Read the model definition and answer for the solid it produces. Units are mm, in the model's axes. A direction names the side the tool comes from. Round coordinates to 2 decimals unless told otherwise and drop trailing zeros. Loops run counter-clockwise (first coordinate to the right, second up) from the corner with the lowest first, then second, coordinate; pieces in that order, holes last. Notation, with made-up numbers: (-13.5, 25.5) - (-7.5, 25.5) arc R9 ccw to (-7.5, 40.5) - close; hole circle Ø8 at (73.25, 39.5). An arc over 180 degrees is marked (long way). Use one line per item in the form item = value. Start each with the question number.
```python
from build123d import *

# Parameters (mm, degrees)
SKETCH1_R           = 3.175
SKETCH1_R_2         = 2.54
BOSS_EXTRUDE1_DEPTH = 3.175
SKETCH2_R           = 11.049
SKETCH2_R_2         = 15.875
SKETCH2_R_3         = 1.27
CUT_EXTRUDE1_DEPTH  = 205.928972451


with BuildPart() as part:
    # Sketch1 → Boss-Extrude1 (new, symmetric)
    with BuildSketch(Plane.XY):
        with BuildLine():
            Line((-83.815331135, 50.8), (83.815331135, 50.8))
            ThreePointArc((83.815331135, 50.8), (193.675, 0), (83.815331135, -50.8))
            Line((83.815331135, -50.8), (-83.815331135, -50.8))
            ThreePointArc((-83.815331135, -50.8), (-193.675, 0), (-83.815331135, 50.8))
        make_face()
        with Locations((-127, 0)):
            Circle(SKETCH1_R, mode=Mode.SUBTRACT)
        with Locations((127, 0)):
            Circle(SKETCH1_R, mode=Mode.SUBTRACT)
        with Locations((-127, 57.15)):
            Circle(SKETCH1_R_2, mode=Mode.SUBTRACT)
        with Locations((-86.588847455, 40.411152545)):
            Circle(SKETCH1_R_2, mode=Mode.SUBTRACT)
        with Locations((-69.85, 0)):
            Circle(SKETCH1_R_2, mode=Mode.SUBTRACT)
        with Locations((-86.588847455, -40.411152545)):
            Circle(SKETCH1_R_2, mode=Mode.SUBTRACT)
        with Locations((-127, -57.15)):
            Circle(SKETCH1_R_2, mode=Mode.SUBTRACT)
        with Locations((-167.411152545, -40.411152545)):
            Circle(SKETCH1_R_2, mode=Mode.SUBTRACT)
        with Locations((-167.411152545, 40.411152545)):
            Circle(SKETCH1_R_2, mode=Mode.SUBTRACT)
        with Locations(Location((127, 57.15, 0), (0, 0, 180))):
            Circle(SKETCH1_R_2, mode=Mode.SUBTRACT)
        with Locations(Location((167.411152545, 40.411152545, 0), (0, 0, 180))):
            Circle(SKETCH1_R_2, mode=Mode.SUBTRACT)
        with Locations(Location((167.411152545, -40.411152545, 0), (0, 0, 180))):
            Circle(SKETCH1_R_2, mode=Mode.SUBTRACT)
        with Locations(Location((127, -57.15, 0), (0, 0, 180))):
            Circle(SKETCH1_R_2, mode=Mode.SUBTRACT)
        with Locations(Location((86.588847455, -40.411152545, 0), (0, 0, 180))):
            Circle(SKETCH1_R_2, mode=Mode.SUBTRACT)
        with Locations(Location((69.85, 0, 0), (0, 0, 180))):
            Circle(SKETCH1_R_2, mode=Mode.SUBTRACT)
        with Locations(Location((86.588847455, 40.411152545, 0), (0, 0, 180))):
            Circle(SKETCH1_R_2, mode=Mode.SUBTRACT)
    extrude(amount=BOSS_EXTRUDE1_DEPTH, both=True)

    # Sketch2 → Cut-Extrude1 (cut, through all)
    with BuildSketch(Plane.XY.offset(3.175)):
        with Locations((-127, 0)):
            Circle(SKETCH2_R)
        with Locations((-155.575, 0)):
            Circle(SKETCH2_R_2)
        with Locations((-155.575, 23.8125)):
            Circle(SKETCH2_R_3)
        with Locations((-138.737019773, 16.837980227)):
            Circle(SKETCH2_R_3)
        with Locations((-138.737019773, -16.837980227)):
            Circle(SKETCH2_R_3)
        with Locations((-155.575, -23.8125)):
            Circle(SKETCH2_R_3)
        with Locations((-172.412980227, -16.837980227)):
            Circle(SKETCH2_R_3)
        with Locations((-179.3875, 0)):
            Circle(SKETCH2_R_3)
        with Locations((-172.412980227, 16.837980227)):
            Circle(SKETCH2_R_3)
        with Locations((-127, 15.875)):
            Circle(SKETCH2_R_3)
        with Locations((-115.774679849, 11.225320151)):
            Circle(SKETCH2_R_3)
        with Locations((-111.125, 0)):
            Circle(SKETCH2_R_3)
        with Locations((-115.774679849, -11.225320151)):
            Circle(SKETCH2_R_3)
        with Locations((-127, -15.875)):
            Circle(SKETCH2_R_3)
        with Locations((-138.225320151, -11.225320151)):
            Circle(SKETCH2_R_3)
        with Locations(Location((138.225320151, 11.225320151, 0), (0, 0, 180))):
            Circle(SKETCH2_R_3)
        with Locations((-138.225320151, 11.225320151)):
            Circle(SKETCH2_R_3)
        with Locations(Location((138.225320151, -11.225320151, 0), (0, 0, 180))):
            Circle(SKETCH2_R_3)
        with Locations(Location((127, -15.875, 0), (0, 0, 180))):
            Circle(SKETCH2_R_3)
        with Locations(Location((115.774679849, -11.225320151, 0), (0, 0, 180))):
            Circle(SKETCH2_R_3)
        with Locations(Location((111.125, 0, 0), (0, 0, 180))):
            Circle(SKETCH2_R_3)
        with Locations(Location((115.774679849, 11.225320151, 0), (0, 0, 180))):
            Circle(SKETCH2_R_3)
        with Locations(Location((127, 15.875, 0), (0, 0, 180))):
            Circle(SKETCH2_R_3)
        with Locations(Location((172.412980227, 16.837980227, 0), (0, 0, 180))):
            Circle(SKETCH2_R_3)
        with Locations(Location((179.3875, 0, 0), (0, 0, 180))):
            Circle(SKETCH2_R_3)
        with Locations(Location((172.412980227, -16.837980227, 0), (0, 0, 180))):
            Circle(SKETCH2_R_3)
        with Locations(Location((155.575, -23.8125, 0), (0, 0, 180))):
            Circle(SKETCH2_R_3)
        with Locations(Location((138.737019773, -16.837980227, 0), (0, 0, 180))):
            Circle(SKETCH2_R_3)
        with Locations(Location((138.737019773, 16.837980227, 0), (0, 0, 180))):
            Circle(SKETCH2_R_3)
        with Locations(Location((155.575, 23.8125, 0), (0, 0, 180))):
            Circle(SKETCH2_R_3)
        with Locations(Location((155.575, 0, 0), (0, 0, 180))):
            Circle(SKETCH2_R_2)
        with Locations(Location((127, 0, 0), (0, 0, 180))):
            Circle(SKETCH2_R)
    extrude(amount=-CUT_EXTRUDE1_DEPTH, mode=Mode.SUBTRACT)


solid = part.part
```
1) A cutting plane is placed at B-B on z = 0.5. Count the separate pieces of the cut face and the enclosed holes in it, plus the area to 3 significant figures.
2) A cutting plane is placed at C-C on y = 29. Write down the section's boundary in (x, z) (3 decimals), plus the area to 3 significant figures.
3) For faces 1 (the flat face through (-1, 50.8, 0)), 2 (the flat face through (1, -50.8, 0)), 3 (the cylindrical face through (168.173, 9.66, 0.044)), determine the directions among +Z, -Z, +X, -X, +Y, -Y from which every point of the face is accessible in a straight line to the end or side of a thin tool.
4) Flat-ended cylindrical pins translate along their axes: pin 1 (1 mm diameter, centred on x = -27, z = 2.5, fed in from +Y); pin 2 (1.5 mm diameter, centred on x = -115.77, y = -11.23, fed in from +Z); pin 3 (1.5 mm diameter, centred on x = -53, z = -2.5, fed in from -Y). Find the tip coordinate at first contact, or state that the pin passes through.
5) A cutting plane is placed at A-A on x = 25.5. Write down the section's boundary in (y, z) (3 decimals).
6) Straight lines are drawn through the part: line 1 (Y direction, x = 127, z = -1.25) (3 decimals); line 2 (X direction, y = -23, z = -2.25); line 3 (Y direction, x = -125.5, z = 1.5). For each, find the intervals that lie inside material, in ascending order. Write a range as from..to.
Checks:
q1.separate_pieces = 1
q1.enclosed_holes = 46
q1.area = 38,900 mm²
q2.outline = (-187.038, -3.175) - (187.038, -3.175) - (187.038, 3.175) - (-187.038, 3.175) - close
q2.area = 2,380 mm²
q3.face_1 = +Z, -Z, +Y
q3.face_2 = +Z, -Z, -Y
q3.face_3 = +Z, -Z
q4.pin_1 = 50.8
q4.pin_2 = through
q4.pin_3 = -50.8
q5.outline = (-50.8, -3.175) - (50.8, -3.175) - (50.8, 3.175) - (-50.8, 3.175) - close
q6.line_1 = -66.675..-59.69, -54.61..-17.145, -14.605..-11.049, 11.049..14.605, 17.145..54.61, 59.69..66.675
q6.line_2 = -189.58..-156.55, -154.6..154.6, 156.55..189.58
q6.line_3 = -66.66..-59.2, -55.1..-10.95, 10.95..55.1, 59.2..66.66
